For this review, take the finished solid that the model builds, in its own axes (mm). Give positions to 0.01 mm unless a question says otherwise; leave off trailing zeros. Order: outer loops, then holes, each group sorted by start corner. A loop starts at its lowest first (then second) coordinate and runs counter-clockwise, first axis right, second up.
from build123d import *

# Parameters (mm, degrees)
BOSS_EXTRUDE1_DEPTH = 0.127


with BuildPart() as part:
    # Sketch1 → Boss-Extrude1 (new body)
    # profile 1 of 5: a face of its own
    with BuildSketch(Plane.XY):
        with BuildLine():
            Line((-0.65, -7.75), (0, -7.75))
            Line((0, -7.75), (0.65, -7.75))
            Line((0.65, -7.75), (0.65, -10.980778661))
            ThreePointArc((0.65, -10.980778661), (8.004686128, -7.544865804), (11, 0))
            ThreePointArc((11, 0), (-7.544865804, 8.004686128), (-0.65, -10.980778661))
            Line((-0.65, -10.980778661), (-0.65, -7.75))
        make_face()
        with BuildLine():
            ThreePointArc((7.75, 0), (5.480077554, -5.480077554), (0, -7.75))
            ThreePointArc((0, -7.75), (-5.480077554, 5.480077554), (7.75, 0))
        make_face(mode=Mode.SUBTRACT)
    # profile 2 of 5: a face of its own
    with BuildSketch(Plane.XY):
        with BuildLine():
            Line((0.65, -7.75), (0, -7.75))
            Line((0, -7.75), (0, -11))
            ThreePointArc((0, -11), (0.325142069, -10.995193615), (0.65, -10.980778661))
            Line((0.65, -10.980778661), (0.65, -7.75))
        make_face()
    # profile 3 of 5: a face of its own
    with BuildSketch(Plane.XY):
        with BuildLine():
            Line((0, -11), (0, -7.75))
            Line((0, -7.75), (-0.65, -7.75))
            Line((-0.65, -7.75), (-0.65, -10.980778661))
            ThreePointArc((-0.65, -10.980778661), (-0.325142069, -10.995193615), (0, -11))
        make_face()
    # profile 4 of 5: a face of its own
    with BuildSketch(Plane.XY):
        with BuildLine():
            Line((0, -15.25), (0, -11))
            ThreePointArc((0, -11), (-0.325142069, -10.995193615), (-0.65, -10.980778661))
            Line((-0.65, -10.980778661), (-0.65, -15.25))
            Line((-0.65, -15.25), (0, -15.25))
        make_face()
    # profile 5 of 5: a face of its own
    with BuildSketch(Plane.XY):
        with BuildLine():
            ThreePointArc((0.65, -10.980778661), (0.325142069, -10.995193615), (0, -11))
            Line((0, -11), (0, -15.25))
            Line((0, -15.25), (0.65, -15.25))
            Line((0.65, -15.25), (0.65, -10.980778661))
        make_face()
    extrude(amount=BOSS_EXTRUDE1_DEPTH)


solid = part.part
1) To check wall thickness, follow line 1 (Y direction, x = 5, z = 0.05); line 2 (X direction, y = -3.25, z = 0.05); line 3 (X direction, y = -12.5, z = 0.05). State the ranges of each line that lie inside material, in increasing order.
Answer sheet:
line 1: y = -9.8 to -5.92, 5.92 to 9.8
line 2: x = -10.51 to -7.04, 7.04 to 10.51
line 3: x = -0.65 to 0.65
2) We need section C-C on y = -12.25. Give the boundary of the cut face in (x, z).
Answer sheet:
outline: (-0.65, 0) - (0.65, 0) - (0.65, 0.13) - (-0.65, 0.13) - close
3) We need section D-D on y = -9.25. Give the boundary of the cut face in (x, z).
Answer sheet:
outline: (-5.95, 0) - (5.95, 0) - (5.95, 0.13) - (-5.95, 0.13) - close
4) We need section B-B on x = -1.75. Give the boundary of the cut face in (y, z).
Answer sheet:
outline: (-10.86, 0) - (-7.55, 0) - (-7.55, 0.13) - (-10.86, 0.13) - close; (7.55, 0) - (10.86, 0) - (10.86, 0.13) - (7.55, 0.13) - close
5) We need section A-A on y = -6.5. Give the boundary of the cut face in (x, z), then the cut area to 3 significant figures.
Answer sheet:
outline: (-8.87, 0) - (-4.22, 0) - (-4.22, 0.13) - (-8.87, 0.13) - close; (4.22, 0) - (8.87, 0) - (8.87, 0.13) - (4.22, 0.13) - close
area: 1.18 mm2
